from build123d import *

# Parameters (mm, degrees)
SKETCH1_W           = 70
SKETCH1_H           = 21.4
BOSS_EXTRUDE1_DEPTH = 5
SKETCH2_W           = 6
SKETCH2_H           = 21.4
SKETCH2_W_2         = 20
CUT_EXTRUDE1_DEPTH  = 3.8
SKETCH3_R           = 1.4
CUT_EXTRUDE2_DEPTH  = 46.232731512


with BuildPart() as part:
    # Sketch1 → Boss-Extrude1 (new body)
    with BuildSketch(Plane.XY):
        with Locations((0, 17.7)):
            Rectangle(SKETCH1_W, SKETCH1_H)
    extrude(amount=BOSS_EXTRUDE1_DEPTH)

    # Sketch2 → Cut-Extrude1 (cut)
    with BuildSketch(Plane.XY.offset(5)):
        with Locations((-32, 17.7)):
            Rectangle(SKETCH2_W, SKETCH2_H)
        with Locations((25, 17.7)):
            Rectangle(SKETCH2_W_2, SKETCH2_H)
    extrude(amount=-CUT_EXTRUDE1_DEPTH, mode=Mode.SUBTRACT)

    # Sketch3 → Cut-Extrude2 (cut, through all)
    with BuildSketch(Plane.XY.offset(1.2)):
        with Locations((32, 23.9)):
            Circle(SKETCH3_R)
        with Locations((-32, 23.9)):
            Circle(SKETCH3_R)
    extrude(amount=-CUT_EXTRUDE2_DEPTH, mode=Mode.SUBTRACT)


solid = part.part
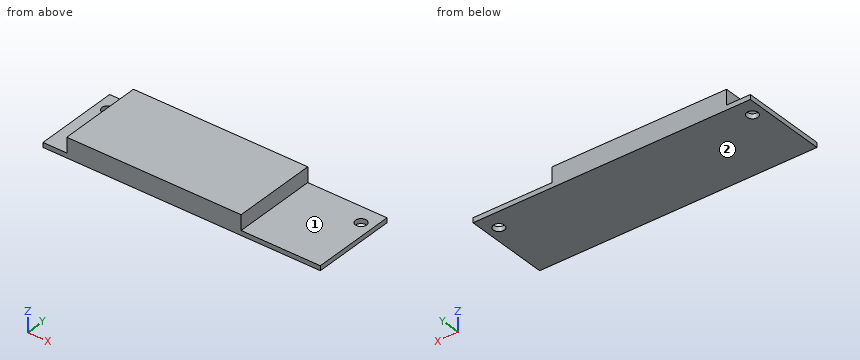
Geometry check sheet. Reference: the model listing, model coordinates, mm. Face numbers are marked on the shaded views. A direction names the side the tool comes from. Round coordinates to 2 decimals unless told otherwise and drop trailing zeros. Loops run counter-clockwise (first coordinate to the right, second up) from the corner with the lowest first, then second, coordinate; pieces in that order, holes last. Notation, with made-up numbers: (79, 5) - (106, 5) arc R12 cw to (106, 24) - close; hole circle Ø2 at (31, -10). An arc over 180 degrees is marked (long way). Answer as CSV lines item,"result".
(1) Cross-section at B-B, the plane y = 23.9. Enter the section's corners in (x, z).
Output values:
outline,"(-35, 0) - (-33.4, 0) - (-33.4, 1.2) - (-35, 1.2) - close; (-30.6, 0) - (30.6, 0) - (30.6, 1.2) - (15, 1.2) - (15, 5) - (-29, 5) - (-29, 1.2) - (-30.6, 1.2) - close; (33.4, 0) - (35, 0) - (35, 1.2) - (33.4, 1.2) - close"
(2) Depth check by flat-ended pin: pin 1 Ø3 at (y, z) = (20, 3.5) entering from -X; pin 2 Ø1.9 at (y, z) = (20, 3.5) entering from +X; pin 3 Ø6 at (x, y) = (30, 15.5) entering from +Z; pin 4 Ø2 at (x, y) = (32, 23.9) entering from +Z. Enter the tip coordinate at first touch or a pass-through.
Output values:
pin 1,"stops at x = -29"
pin 2,"stops at x = 15"
pin 3,"stops at z = 1.2"
pin 4,"passes through"
(3) Set-up check for the marked faces 1 and 2: record each of +Z, -Z, +X, -X, +Y, -Y from which the full face is reachable in a straight line by a thin tool's end or side.
Output values:
face 1,"+Z, +X, +Y, -Y"
face 2,"-Z, +X, -X, +Y, -Y"
(4) Material ranges on line 1 along Y through (x, z) = (32, 0.9); line 2 along X through (y, z) = (15, 2.05); line 3 along Z through (x, y) = (21, 13.5), recorded low to high.
Output values:
line 1,"y = 7 to 22.5, 25.3 to 28.4"
line 2,"x = -29 to 15"
line 3,"z = 0 to 1.2"
(5) Cross-section at A-A, the plane x = 32. Enter the section's corners in (y, z), and give its area (3 significant figures).
Output values:
outline,"(7, 0) - (22.5, 0) - (22.5, 1.2) - (7, 1.2) - close; (25.3, 0) - (28.4, 0) - (28.4, 1.2) - (25.3, 1.2) - close"
area,"22.3 mm²"
(6) Cross-section at C-C, the plane y = 10.75. Enter the section's corners in (x, z).
Output values:
outline,"(-35, 0) - (35, 0) - (35, 1.2) - (15, 1.2) - (15, 5) - (-29, 5) - (-29, 1.2) - (-35, 1.2) - close"
(7) Cross-section at D-D, the plane x = 16. Enter the section's corners in (y, z).
Output values:
outline,"(7, 0) - (28.4, 0) - (28.4, 1.2) - (7, 1.2) - close"
